from build123d import *

# Parameters (mm, degrees)
CROQUIS1_R              = 2.2
SALIENTE_EXTRUIR1_DEPTH = 1.6
SALIENTE_EXTRUIR3_START = -2
CROQUIS3_W              = 12
CROQUIS3_H              = 6.7
CROQUIS3_W_2            = 11
CROQUIS3_H_2            = 5.7
SALIENTE_EXTRUIR3_DEPTH = 6


with BuildPart() as part:
    # Croquis1 → Saliente-Extruir1 (new body)
    with BuildSketch(Plane.XY):
        with BuildLine():
            Line((7.4, -12.85), (-7.4, -12.85))
            Line((-7.4, -12.85), (-7.4, 7.05))
            ThreePointArc((-7.4, 7.05), (-6.2, 8.25), (-7.4, 9.45))
            Line((-7.4, 9.45), (-7.4, 12.85))
            Line((-7.4, 12.85), (7.4, 12.85))
            Line((7.4, 12.85), (7.4, 9.45))
            ThreePointArc((7.4, 9.45), (6.2, 8.25), (7.4, 7.05))
            Line((7.4, 7.05), (7.4, -12.85))
        make_face()
        with Locations((0, 9.65)):
            Circle(CROQUIS1_R, mode=Mode.SUBTRACT)
    extrude(amount=SALIENTE_EXTRUIR1_DEPTH)

    # Croquis3 → Saliente-Extruir3 (add)
    with BuildSketch(Plane.XZ.offset(12.85).offset(SALIENTE_EXTRUIR3_START)):
        with Locations((0, 4.95)):
            Rectangle(CROQUIS3_W, CROQUIS3_H)
        with Locations((0, 4.95)):
            Rectangle(CROQUIS3_W_2, CROQUIS3_H_2, mode=Mode.SUBTRACT)
    extrude(amount=-SALIENTE_EXTRUIR3_DEPTH)


solid = part.part
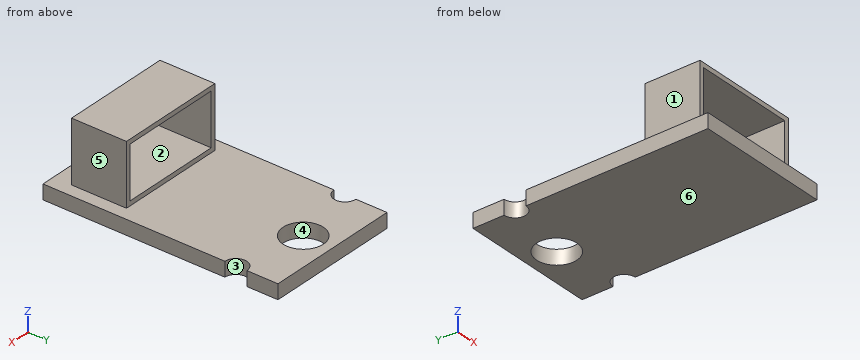
Could you check a few things on this model? Use its own coordinates, in mm. Face numbers are marked on the shaded views. A direction names the side the tool comes from. Give positions to 0.01 mm unless a question says otherwise; leave off trailing zeros. Order: outer loops, then holes, each group sorted by start corner. A loop starts at its lowest first (then second) coordinate and runs counter-clockwise, first axis right, second up. Notation, with made-up numbers: (32.25, -20) - (36.25, -20) arc R20 cw to (36.25, 13) - close; hole circle Ø9 at (22, -32). An arc over 180 degrees is marked (long way). Return JSON: item names as keys, results as strings. Group by question number.
Q1. Suppose I cut it at B-B, the plane x = 0. Please give me the cut outline in (y, z), and give its area (3 significant figures).
Q2. Thinking about a two-plate mould opening in X: for the marked faces 4, 5 and 6, which applies, pulls with the +X half, pulls with the -X half, needs draft (parallel to the pull), parting line crosses it, or undercut?
Q3. Suppose I cut it at C-C, the plane y = 8.25. Please give me the cut outline in (x, z), and give its area (3 significant figures).
Q4. Will these pins go through, and if not, where does the flat tip stop? pin 1 Ø1.7 at (y, z) = (-7.5, 6) entering from -X; pin 2 Ø1.5 at (x, y) = (-4.5, 7) entering from -Z; pin 3 Ø5.5 at (x, y) = (0, 9.65) entering from +Z; pin 4 Ø1.5 at (y, z) = (9, 4) entering from +X.
Q5. Suppose I cut it at A-A, the plane z = 6.25. Please give me the cut outline in (x, y), and give its area (3 significant figures).
Q6. Suppose I cut it at D-D, the plane z = 0.5. Please give me the cut outline in (x, y), and give its area (3 significant figures).
Q7. Which directions (+Z, -Z, +X, -X, +Y, -Y) give clear straight access to the entire face, cutting with the end or side of a thin tool? Please do the marked faces 1, 2 and 3.
Q8. Please list where these lines run through material, in increasing order: line 1 along Y through (x, z) = (0, 1.35); line 2 along Z through (x, y) = (-2.25, -5.75); line 3 along Z through (x, y) = (5.5, 4.25). Write a range as [from, to].
Resolved:
{
 "1": {"outline": "(-12.85, 0) - (7.45, 0) - (7.45, 1.6) - (-4.85, 1.6) - (-4.85, 2.1) - (-10.85, 2.1) - (-10.85, 1.6) - (-12.85, 1.6) - close; (-10.85, 7.8) - (-4.85, 7.8) - (-4.85, 8.3) - (-10.85, 8.3) - close; (11.85, 0) - (12.85, 0) - (12.85, 1.6) - (11.85, 1.6) - close", "area": "40.1 mm2"},
 "2": {"face 4": "undercut", "face 5": "pulls with the +X half", "face 6": "needs draft"},
 "3": {"outline": "(-6.2, 0) - (-1.7, 0) - (-1.7, 1.6) - (-6.2, 1.6) - close; (1.7, 0) - (6.2, 0) - (6.2, 1.6) - (1.7, 1.6) - close", "area": "14.4 mm2"},
 "4": {"pin 1": "stops at x = -6", "pin 2": "stops at z = 0", "pin 3": "stops at z = 1.6", "pin 4": "passes through"},
 "5": {"outline": "(-6, -10.85) - (-5.5, -10.85) - (-5.5, -4.85) - (-6, -4.85) - close; (5.5, -10.85) - (6, -10.85) - (6, -4.85) - (5.5, -4.85) - close", "area": "6.00 mm2"},
 "6": {"outline": "(-7.4, -12.85) - (7.4, -12.85) - (7.4, 7.05) arc R1.2 cw to (7.4, 9.45) - (7.4, 12.85) - (-7.4, 12.85) - (-7.4, 9.45) arc R1.2 cw to (-7.4, 7.05) - close; hole circle Ø4.4 at (0, 9.65)", "area": "361 mm2"},
 "7": {"face 1": "+Z, -X, +Y, -Y", "face 2": "+Y, -Y", "face 3": "+Z, -Z, +X"},
 "8": {"line 1": "y = [-12.85, 7.45], [11.85, 12.85]", "line 2": "z = [0, 2.1], [7.8, 8.3]", "line 3": "z = [0, 1.6]"}
}
